Input: dimensioned drawing with shaded views. Units: mm. Origin: part minimum x, y, z. Give positions to 0.01 mm unless a question says otherwise; leave off trailing zeros. Order: outer loops, then holes, each group sorted by start corner. A loop starts at its lowest first (then second) coordinate and runs counter-clockwise, first axis right, second up.
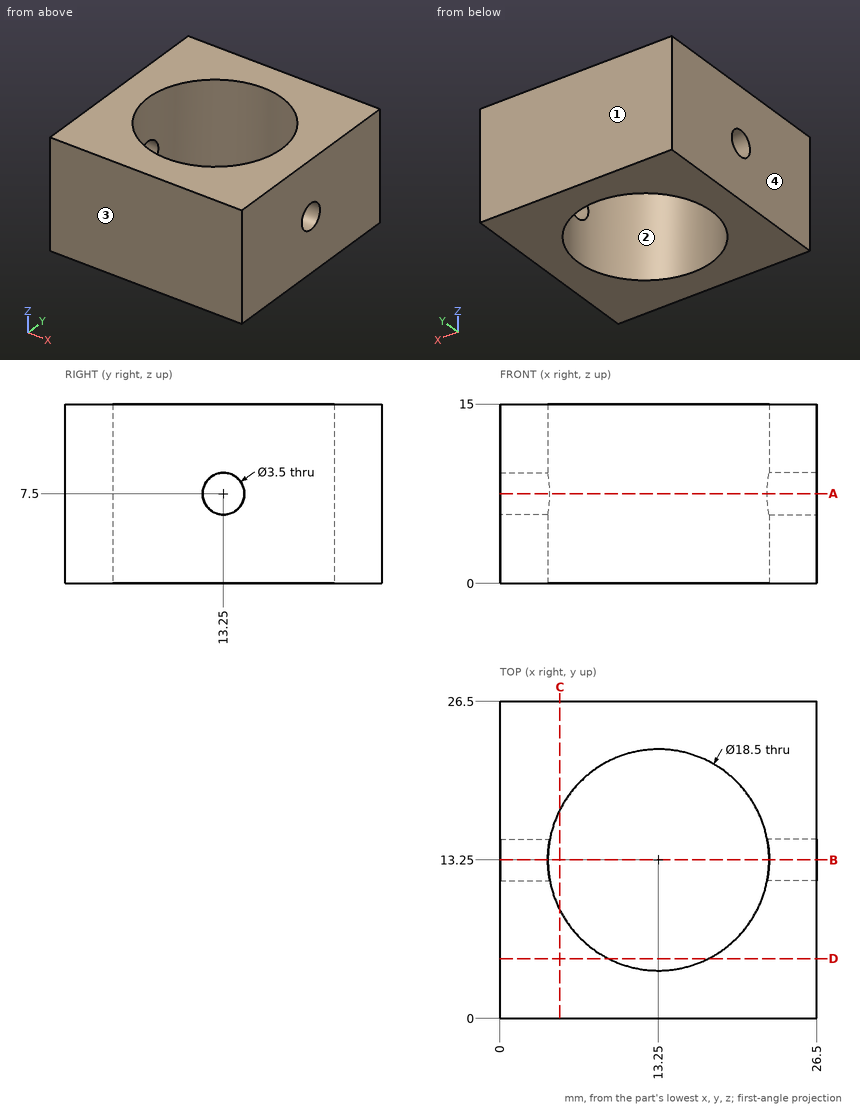
1) Section query C-C, the plane x = 5. Return the cut outline in (y, z).
Report:
outline: (0, 0) - (9.07, 0) - (9.07, 15) - (0, 15) - close; (17.43, 0) - (26.5, 0) - (26.5, 15) - (17.43, 15) - close
2) Draft query along Y for the marked faces 1, 2, 3 and 4. Return one class per face: +Y half, -Y half, draft (parallel to the pull), parting line (faces both ways), or undercut.
Report:
face 1: +Y half
face 2: undercut
face 3: -Y half
face 4: draft
3) Section query B-B, the plane y = 13.25. Return the cut outline in (x, z).
Report:
outline: (0, 0) - (4, 0) - (4, 5.75) - (0, 5.75) - close; (0, 9.25) - (4, 9.25) - (4, 15) - (0, 15) - close; (22.5, 0) - (26.5, 0) - (26.5, 5.75) - (22.5, 5.75) - close; (22.5, 9.25) - (26.5, 9.25) - (26.5, 15) - (22.5, 15) - close
4) Section query A-A, the plane z = 7.5. Return the cut outline in (x, y).
Report:
outline: (0, 0) - (26.5, 0) - (26.5, 11.5) - (22.33, 11.5) arc R9.25 cw to (4.17, 11.5) - (0, 11.5) - close; (0, 15) - (4.17, 15) arc R9.25 cw to (22.33, 15) - (26.5, 15) - (26.5, 26.5) - (0, 26.5) - close
5) Material intervals for L1, parallel to Y at x = 13.25, z = 4; L2, parallel to Y at x = 24.15, z = 7.5, sorted ascending.
Report:
L1: y = 0 to 4, 22.5 to 26.5
L2: y = 0 to 11.5, 15 to 26.5
